```python
from build123d import *

# Parameters (mm, degrees)
CUT_EXTRUDE1_START = -80
SKETCH6_R          = 2
CUT_EXTRUDE1_DEPTH = 68.253319148
SKETCH7_R          = 3
CUT_EXTRUDE2_DEPTH = 149.969232185
CIRPATTERN1_COUNT  = 6


with BuildPart() as part:
    # Sketch1 → Revolve1 (revolve)
    with BuildSketch(Plane(origin=(0, 0, 0), x_dir=(0, 0, -1), z_dir=(1, 0, 0)), mode=Mode.PRIVATE) as revolve1_sk:
        with BuildLine():
            Line((64.8, 0), (-64.8, 0))
            ThreePointArc((-64.8, 0), (-53.198891339, 36.998891339), (-22.549445669, 60.75))
            Line((-22.549445669, 60.75), (-9.19, 60.75))
            Line((-9.19, 60.75), (-9.19, 80))
            Line((-9.19, 80), (-3.79, 80))
            Line((-3.79, 80), (-3.79, 93.5))
            Line((-3.79, 93.5), (3.81, 93.5))
            Line((3.81, 93.5), (3.81, 84))
            Line((3.81, 84), (11.41, 84))
            Line((11.41, 84), (11.41, 70))
            Line((11.41, 70), (16.31, 70))
            Line((16.31, 70), (16.31, 60.75))
            Line((16.31, 60.75), (22.549445669, 60.75))
            ThreePointArc((22.549445669, 60.75), (53.198891339, 36.998891339), (64.8, 0))
        make_face()
    revolve(revolve1_sk.sketch.rotate(Axis((0, 0, 0), (0, 0, -1)), 90), axis=Axis((0, 0, 0), (0, 0, -1)))

    # Sketch6 → Cut-Extrude1 (cut, through all)
    with BuildSketch(Plane(origin=(0, 0, 0), x_dir=(0, 0, -1), z_dir=(1, 0, 0)).offset(CUT_EXTRUDE1_START)):
        Circle(SKETCH6_R)
    cut_extrude1 = extrude(amount=-CUT_EXTRUDE1_DEPTH, mode=Mode.SUBTRACT)

    # Sketch7 → Cut-Extrude2 (cut, through all)
    with BuildSketch(Plane(origin=(0, 0, -3.81), x_dir=(-1, 0, 0), z_dir=(0, 0, -1))):
        with Locations((0, 88.5)):
            Circle(SKETCH7_R)
    cut_extrude2 = extrude(amount=-CUT_EXTRUDE2_DEPTH, mode=Mode.SUBTRACT)

    # CirPattern1: Cut-Extrude1, Cut-Extrude2 ×6 about axis
    cirpattern1_axis = Axis((0, 0, 0), (0, 0, 1))
    add([cut_extrude1.rotate(cirpattern1_axis, i * 360 / CIRPATTERN1_COUNT) for i in range(1, CIRPATTERN1_COUNT)], mode=Mode.SUBTRACT)
    add([cut_extrude2.rotate(cirpattern1_axis, i * 360 / CIRPATTERN1_COUNT) for i in range(1, CIRPATTERN1_COUNT)], mode=Mode.SUBTRACT)


solid = part.part
```
Design review of the part built by this model. Coordinates are the model's own, in mm. A direction names the side the tool comes from. Coordinates: 2 decimals unless noted, no trailing zeros. Order: outer loops, then holes, each group sorted by start corner. A loop starts at its lowest first (then second) coordinate and runs counter-clockwise, first axis right, second up.
1) Take a section at B-B, the plane x = -55.5. Give the boundary of the cut face in (y, z), and give its area (3 significant figures).
2) Take a section at A-A, the plane y = -88.5. Give the boundary of the cut face in (x, z), and give its area (3 significant figures).
3) Mouldability with a two-part tool opening along X and no side actions: class faces 1 (the cylindrical face through (0.65, 85.57, -0.06)), 2 (the cylindrical face through (80.12, -25.23, -7.66)), 3 (the flat face through (-41, 69, 3.79)) as +X half, -X half, draft (parallel to the pull), parting line (faces both ways), or undercut.
4) Wall thickness on line 1 along X through (y, z) = (44, -1); line 2 along X through (y, z) = (70.5, -1); line 3 along Z through (x, y) = (7, 85): over which ranges is each line inside the solid? List them lowest first.
5) For faces 4 (the flat face through (-21.1, -57.4, -16.31)), 5 (the cylindrical face through (28.032, 53.896, 15.776)), 6 (the cylindrical face through (78.256, 41.72, -0.063)), list the 3-axis set-ups (+Z, -Z, +X, -X, +Y, -Y) from which the entire face can be reached by the end or side of a thin tool; tool diameter is ignored.
6) Clearance check with flat-ended pins moving along their axes: pin 1 (10 mm diameter, centred on y = -18.5, z = 33.5, fed in from +X); pin 2 (1.5 mm diameter, centred on x = 24, y = -33.5, fed in from +Z); pin 3 (1.2 mm diameter, centred on y = 0, z = -1, fed in from +X); pin 4 (3.5 mm diameter, centred on x = 76.64, y = 44.25, fed in from -Z). State where each tip first meets the part, or that it passes through.
7) Take a section at C-C, the plane y = 44.25. State how many separate pieces and enclosed holes the cut face has, and give its area (3 significant figures).
8) Take a section at D-D, the plane y = -23.5. Give the boundary of the cut face in (x, z), and give its area (3 significant figures).
Returned:
1. outline: (-75.25, -3.81) - (-63.05, -3.81) - (-63.05, -11.41) - (-42.66, -11.41) - (-42.66, -16.31) - (-24.7, -16.31) - (-24.7, -22.55) arc R33.45 ccw to (24.7, -22.55) - (24.7, -16.31) - (42.66, -16.31) - (42.66, -11.41) - (63.05, -11.41) - (63.05, -3.81) - (75.25, -3.81) - (75.25, 3.79) - (57.62, 3.79) - (57.62, 9.19) - (24.7, 9.19) - (24.7, 22.55) arc R33.45 ccw to (-24.7, 22.55) - (-24.7, 9.19) - (-57.62, 9.19) - (-57.62, 3.79) - (-75.25, 3.79) - close
1. area: 4,860 mm2
2. outline: (-30.17, -3.81) - (-3, -3.81) - (-3, 3.79) - (-30.17, 3.79) - close; (3, -3.81) - (30.17, -3.81) - (30.17, 3.79) - (3, 3.79) - close
2. area: 413 mm2
3. face 1: undercut
3. face 2: parting line
3. face 3: draft
4. line 1: x = -82.5 to -79.63, -73.65 to 73.65, 79.63 to 82.5
4. line 2: x = -61.42 to -42.7, -38.7 to 38.7, 42.7 to 61.42
4. line 3: z = -3.81 to 3.79
5. face 4: -Z
5. face 5: +Z
5. face 6: +Z, -Z
6. pin 1: stops at x = 55.61
6. pin 2: stops at z = 50.62
6. pin 3: stops at x = 80
6. pin 4: passes through
7. separate pieces: 3
7. enclosed holes: 0
7. area: 8,070 mm2
8. outline: (-90.5, -3.81) - (-80.65, -3.81) - (-80.65, -11.41) - (-65.94, -11.41) - (-65.94, -16.31) - (-56.02, -16.31) - (-56.02, -22.55) arc R60.39 ccw to (56.02, -22.55) - (56.02, -16.31) - (65.94, -16.31) - (65.94, -11.41) - (80.65, -11.41) - (80.65, -3.81) - (90.5, -3.81) - (90.5, 3.79) - (76.47, 3.79) - (76.47, 9.19) - (56.02, 9.19) - (56.02, 22.55) arc R60.39 ccw to (-56.02, 22.55) - (-56.02, 9.19) - (-76.47, 9.19) - (-76.47, 3.79) - (-90.5, 3.79) - close
8. area: 12,400 mm2
